Autodesk Fusion 360 part; units mm, degrees
sketch "Sketch1" plane through (0, 0, 0) normal (0, 1, 0) x (1, 0, 0)
  line L0 (0, -20) -> (100, -20)
  line L1 (100, -20) -> (100, 0)
  line L2 (100, 0) -> (0, 0)
  line L3 (0, 0) -> (0, -20)
  dimension "d1" = 100
extrude "Extrude1" add sketch "Sketch1" along normal blind 2
sketch "Sketch2" plane through (0, 0, 0) normal (0, 1, 0) x (1, 0, 0)
  circle A0 centre (14, -10) radius 1.5
  dimension "d4" = 3
extrude "Extrude2" add sketch "Sketch2" against normal blind 5
sketch "Sketch3" plane through (0, 0, 0) normal (0, 1, 0) x (1, 0, 0)
  circle A0 centre (86, -10) radius 1.5
  dimension "d7" = 3
extrude "Extrude3" add sketch "Sketch3" against normal blind 5
fillet "Fillet1" radius 5 1 edges at (0, 1, 20)
fillet "Fillet2" radius 5 1 edges at (100, 1, 20)
fillet "Fillet3" radius 5 1 edges at (100, 1, 0)
fillet "Fillet4" radius 5 1 edges at (0, 1, 0)
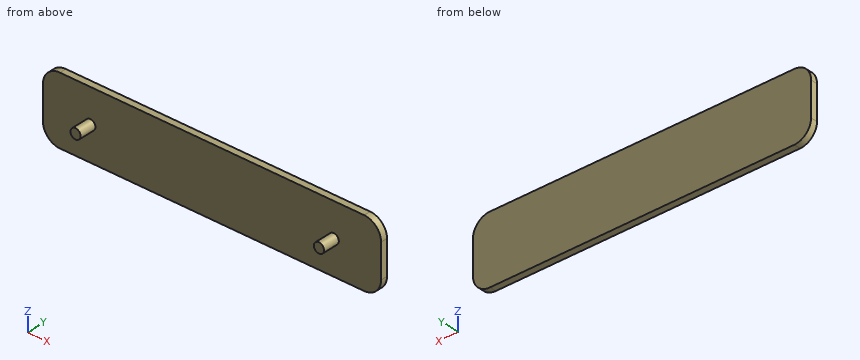
Work out the finished part from the listing and answer in its coordinate system (mm). Give positions to 0.01 mm unless a question says otherwise; leave off trailing zeros. Loops run counter-clockwise (first coordinate to the right, second up) from the corner with the lowest first, then second, coordinate; pieces in that order, holes last. Notation, with made-up numbers: (11, 30.25) - (33, 30.25) arc R20 ccw to (33, 46.25) - close; hole circle Ø4 at (63.25, 31). An arc over 180 degrees is marked (long way). Answer in a Markdown table with one row per item. Add a question column.
Q1. This flat-tipped pin is pushed along its axis until it touches: P1, Ø10, axis at x = 46.5, z = 10.5, coming from the -Y side. Where does it stop, or does it pass through?
Q2. Consider line 1 along Y through (x, z) = (53, 2.5); line 2 along X through (y, z) = (-0.75, 10.5); line 3 along X through (y, z) = (1.5, 16.5). Determine where each line is inside the solid, lowest interval first.
Q3. The part is cut by section C-C (y = -3). Determine the outline of the cut face in (x, z).
Q4. The part is cut by section A-A (x = 86). Determine the outline of the cut face in (y, z), and give its area (3 significant figures).
Q5. The part is cut by section B-B (z = 10). Determine the outline of the cut face in (x, y), and give its area (3 significant figures).
Q6. The part is cut by section D-D (x = 76). Determine the outline of the cut face in (y, z), and give its area (3 significant figures).
Solution:
| question | item | result |
|---|---|---|
| 1 | P1 | stops at y = 0 |
| 2 | line 1 | y = 0 to 2 |
| 2 | line 2 | x = 12.59 to 15.41, 84.59 to 87.41 |
| 2 | line 3 | x = 0.23 to 99.77 |
| 3 | outline | circle Ø3 at (14, 10); circle Ø3 at (86, 10) |
| 4 | outline | (-5, 8.5) - (0, 8.5) - (0, 0) - (2, 0) - (2, 20) - (0, 20) - (0, 11.5) - (-5, 11.5) - close |
| 4 | area | 55.0 mm² |
| 5 | outline | (0, 0) - (12.5, 0) - (12.5, -5) - (15.5, -5) - (15.5, 0) - (84.5, 0) - (84.5, -5) - (87.5, -5) - (87.5, 0) - (100, 0) - (100, 2) - (0, 2) - close |
| 5 | area | 230 mm² |
| 6 | outline | (0, 0) - (2, 0) - (2, 20) - (0, 20) - close |
| 6 | area | 40.0 mm² |
